```python
from build123d import *

# Parameters (mm, degrees)
STOCK_POST_1_START     = -5
STOCK_POST_1_OUTLINE_W = 200
STOCK_POST_1_OUTLINE_H = 150
STOCK_POST_1_DEPTH     = 5
F_12_0MM_DOWEL_HOLE1_D = 12


# Read off the part's stored shape, not the designer's step: Stock-Post-1
with BuildPart() as part:
    # Stock-Post-1 outline → Stock-Post-1 (new body)
    with BuildSketch(Plane.XY.offset(STOCK_POST_1_START)):
        with Locations((50, 25)):
            Rectangle(STOCK_POST_1_OUTLINE_W, STOCK_POST_1_OUTLINE_H)
    extrude(amount=STOCK_POST_1_DEPTH)

    # Ø12.0mm Dowel Hole1 (through all)
    with Locations(Plane.XY):
        with Locations((-30, -30), (-30, 80), (130, 80), (130, -30)):
            Hole(F_12_0MM_DOWEL_HOLE1_D / 2)


solid = part.part
```
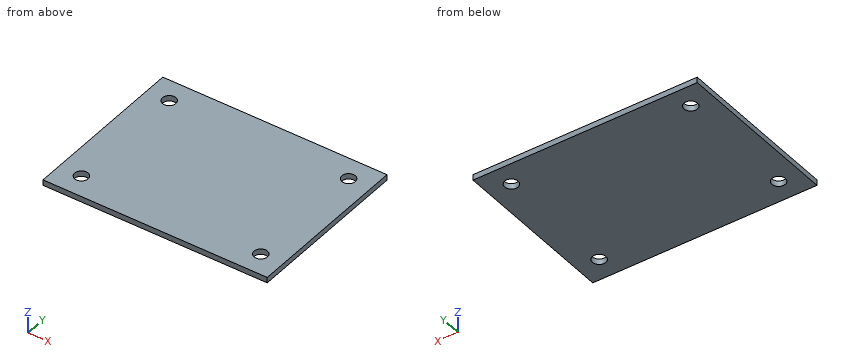
Source: CAD feature listing. Evaluate the final solid. Frame: model axes, mm. Coordinates: 2 decimals unless noted, no trailing zeros. Write each loop counter-clockwise with the first axis right and the second up, starting at its lowest first coordinate (ties: lowest second). Pieces come first, ordered by that corner, then holes. Notation, with made-up numbers: (68, 8) -> (123, 8) arc R20 cw to (123, 44) -> close; hole circle Ø11 at (80.25, 23). An arc over 180 degrees is marked (long way). Return JSON: item names as keys, results as strings. Group by question number.
1) Section query A-A, the plane y = -30. Return loops of the section in (x, z), plus the area to 3 significant figures.
2) Ray query, line 1 along Y through (x, z) = (130, -2); line 2 along Y through (x, z) = (-28, -2.5); line 3 along X through (y, z) = (-27, -2.05). Return the intervals inside material, ascending.
3) Section query B-B, the plane z = -1.6. Return loops of the section in (x, y).
4) Section query C-C, the plane x = 130. Return loops of the section in (y, z).
From the geometry:
{
 "1": {"outline": "(-50, -5) -> (-36, -5) -> (-36, 0) -> (-50, 0) -> close; (-24, -5) -> (124, -5) -> (124, 0) -> (-24, 0) -> close; (136, -5) -> (150, -5) -> (150, 0) -> (136, 0) -> close", "area": "880 mm²"},
 "2": {"line 1": "-50 to -36, -24 to 74, 86 to 100", "line 2": "-50 to -35.66, -24.34 to 74.34, 85.66 to 100", "line 3": "-50 to -35.2, -24.8 to 124.8, 135.2 to 150"},
 "3": {"outline": "(-50, -50) -> (150, -50) -> (150, 100) -> (-50, 100) -> close; hole circle Ø12 at (-30, -30); hole circle Ø12 at (-30, 80); hole circle Ø12 at (130, -30); hole circle Ø12 at (130, 80)"},
 "4": {"outline": "(-50, -5) -> (-36, -5) -> (-36, 0) -> (-50, 0) -> close; (-24, -5) -> (74, -5) -> (74, 0) -> (-24, 0) -> close; (86, -5) -> (100, -5) -> (100, 0) -> (86, 0) -> close"}
}
